Could you check a few things on this model? Use its own coordinates, in mm. A direction names the side the tool comes from. Give positions to 0.01 mm unless a question says otherwise; leave off trailing zeros. Loops run counter-clockwise (first coordinate to the right, second up) from the corner with the lowest first, then second, coordinate; pieces in that order, holes last. Notation, with made-up numbers: (41.5, 9.25) - (54.5, 9.25) arc R18 ccw to (54.5, 23.25) - close; hole circle Ø6 at (89.5, 41). An arc over 180 degrees is marked (long way). One line per item, written item: value. Start each with the question number.
Q1. I want a section at B-B (y = -7). Please give me the cut outline in (x, z), then the cut area to 3 significant figures.
Q2. If we mould it in two halves opening along Y, with no side actions, what happens to faces 1 (the face through (21.581, -3.647, 1.24)), 2 (the face through (2.655, -10.611, 52.958)), 3 (the face through (16, -11, 0))? For each: released by +Y, released by -Y, zero draft, split by the parting line, or undercut.
Q3. I want a section at D-D (y = 6). Please give me the cut outline in (x, z), then the cut area to 3 significant figures.
Q4. For faces 4 (the face through (21, -6, 56)), 5 (the face through (21.463, -6.503, 24.65)), which set-ups out of +Z, -Z, +X, -X, +Y, -Y let a thin tool reach every point of the face, with its end or its side?
Q5. If I drill on line 1 (X direction, y = -2.5, z = 3); line 2 (Y direction, x = 21.35, z = 1); line 3 (X direction, y = -1.75, z = 40), over which ranges is the centre line in solid material (lowest first)? Write a range as from..to.
Q6. I want a section at C-C (z = 1). Please give me the cut outline in (x, y), then the cut area to 3 significant figures.
Q7. I want a section at A-A (x = 18.5). Please give me the cut outline in (y, z), then the cut area to 3 significant figures.
Q8. I'm going to push flat-ended pins straight in: P1, Ø6, axis at x = 6.5, z = 39.5, coming from the -Y side; P2, Ø6, axis at x = 9, y = -4, coming from the +Z side; P3, Ø1.5, axis at y = 6.5, z = 7.5, coming from the +X side; P4, Ø4, axis at x = 18.5, z = 20, coming from the -Y side. Where does each tip first touch, or does it pass through?
```python
from build123d import *

# Parameters (mm, degrees)
SKETCH1_R             = 9.45
SKETCH1_R_2           = 8.3
BOSS_EXTRUDE1_DEPTH   = 50
SKETCH2_R             = 12.7
SKETCH2_R_2           = 8.3
BOSS_EXTRUDE2_DEPTH   = 6
M2X0_4_TAPPED_HOLE1_D = 1.6


with BuildPart() as part:
    # Sketch1 → Boss-Extrude1 (new body)
    with BuildSketch(Plane.XY):
        with Locations((12.733633013, -2.883668241)):
            Circle(SKETCH1_R)
        with Locations((12.733633013, -2.883668241)):
            Circle(SKETCH1_R_2, mode=Mode.SUBTRACT)
    extrude(amount=BOSS_EXTRUDE1_DEPTH)

    # Sketch2 → Boss-Extrude2 (add)
    with BuildSketch(Plane.XY.offset(50)):
        with Locations((12.733633013, -2.883668241)):
            Circle(SKETCH2_R)
        with Locations((12.733633013, -2.883668241)):
            Circle(SKETCH2_R_2, mode=Mode.SUBTRACT)
    extrude(amount=BOSS_EXTRUDE2_DEPTH)

    # M2x0.4 Tapped Hole1 (through all)
    with Locations(Plane(origin=(22.183633013, -2.883668241, 1), x_dir=(0, 1, 0), z_dir=(1, 0, 0))):
        with Locations((0, 0)):
            Hole(M2X0_4_TAPPED_HOLE1_D / 2)


solid = part.part
```
Worked answers:
1. outline: (0.72, 50) - (4.23, 50) - (4.23, 0) - (5.53, 0) - (5.53, 56) - (0.72, 56) - close; (19.94, 0) - (21.24, 0) - (21.24, 50) - (24.75, 50) - (24.75, 56) - (19.94, 56) - close
1. area: 188 mm²
2. face 1: undercut
2. face 2: split by the parting line
2. face 3: zero draft
3. outline: (3.66, 50) - (9.51, 50) - (9.51, 0) - (15.96, 0) - (15.96, 50) - (21.81, 50) - (21.81, 56) - (3.66, 56) - close
3. area: 431 mm²
4. face 4: +Z, +X, -X, +Y, -Y
4. face 5: -Z
5. line 1: x = 3.29..4.44, 21.02..22.18
5. line 2: y = -6.76..-3.68, -2.08..1
5. line 3: x = 3.35..4.51, 20.96..22.12
6. outline: (3.32, -3.68) arc R9.45 ccw to (22.15, -3.68) - (20.99, -3.68) arc R8.3 cw to (4.47, -3.68) - close; (3.32, -2.08) - (4.47, -2.08) arc R8.3 cw to (20.99, -2.08) - (22.15, -2.08) arc R9.45 ccw to start
6. area: 60.4 mm²
7. outline: (-14.2, 50) - (-10.37, 50) - (-10.37, 0) - (-8.85, 0) - (-8.85, 56) - (-14.2, 56) - close; (3.09, 0) - (4.6, 0) - (4.6, 50) - (8.43, 50) - (8.43, 56) - (3.09, 56) - close
7. area: 216 mm²
8. P1: stops at y = -11.76
8. P2: passes through
8. P3: stops at x = 16.58
8. P4: stops at y = -11.55
